Read the model definition and answer for the solid it produces. Units are mm, in the model's axes. Face numbers are marked on the shaded views. A direction names the side the tool comes from. Round coordinates to 2 decimals unless told otherwise and drop trailing zeros. Loops run counter-clockwise (first coordinate to the right, second up) from the corner with the lowest first, then second, coordinate; pieces in that order, holes last. Notation, with made-up numbers: M -5.5,47 L 23.5,47 A23 cw 23.5,78 Z; hole C 44.25,52.25 d5. An arc over 180 degrees is marked long. Write each question's results on one line, items separated by ' | '.
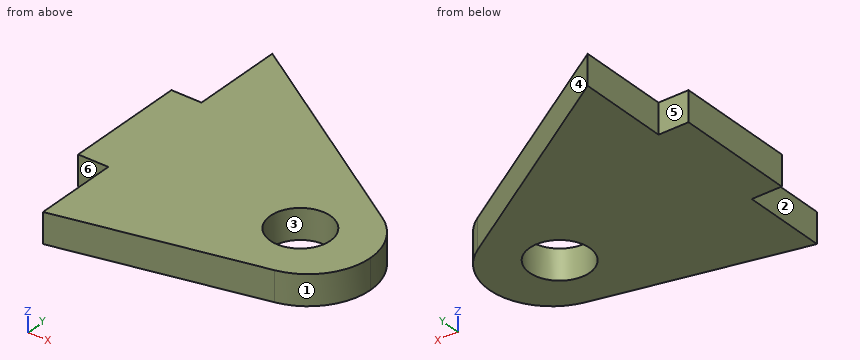
from build123d import *

# Parameters (mm, degrees)
SKETCH1_W                   = 68.548183611
SKETCH1_H                   = 64.912098736
BOSS_EXTRUDE1_DEPTH         = 3.175
F_1_4_0_25_DIAMETER_HOLE1_D = 6.35
CUT_EXTRUDE1_DEPTH          = 95.459063428
FILLET1_R                   = 6.604
SKETCH5_W                   = 3.175
SKETCH5_H                   = 12.7
BOSS_EXTRUDE2_DEPTH         = 3.175


with BuildPart() as part:
    # Sketch1 → Boss-Extrude1 (new body)
    with BuildSketch(Plane.XY):
        with Locations((34.274091805, 32.456049368)):
            Rectangle(SKETCH1_W, SKETCH1_H)
    extrude(amount=BOSS_EXTRUDE1_DEPTH)

    # 1/4 (0.25) Diameter Hole1 (through all)
    with Locations(Plane(origin=(0, 0, 0), x_dir=(-1, 0, 0), z_dir=(0, 0, -1))):
        with Locations((-18.542, 44.846098736)):
            Hole(F_1_4_0_25_DIAMETER_HOLE1_D / 2)

    # Sketch4 → Cut-Extrude1 (cut, through all)
    with BuildSketch(Plane(origin=(0, 0, 0), x_dir=(-1, 0, 0), z_dir=(0, 0, -1))):
        Polygon((-26.0096, 48.402098736), (0, 64.912098736), (-68.548183611, 64.912098736), (-68.548183611, 0), (0, 0), (0, 33.670098736), (-26.0096, 39.512098736), align=None)
    extrude(amount=-CUT_EXTRUDE1_DEPTH, mode=Mode.SUBTRACT)

    # Fillet1
    # the kernel refuses this fillet: 6.604 mm, written as the material it takes off along each edge
    with BuildSketch(Plane(origin=(26.0096, 48.402098736, -9.075328034), x_dir=(-0.84427202966114, 0.5359148625778718, 0), z_dir=(0, 0, 1))) as fillet1_piece_1:
        with BuildLine():
            CenterArc((FILLET1_R * 0.549686737352, FILLET1_R), FILLET1_R, 212.405976432, 57.594023568)
            Line((-FILLET1_R * 0.294585292309, FILLET1_R * 0.464085137422), (0, 0))
            Line((0, 0), (FILLET1_R * 0.549686737352, 0))
        make_face()
    extrude(amount=21.325656067, mode=Mode.SUBTRACT)
    with BuildSketch(Plane(origin=(26.0096, 39.512098736, -13.213034706), x_dir=(-0.9756913106586464, -0.21914941547997013, 0), z_dir=(0, 0, 1))) as fillet1_piece_2:
        with BuildLine():
            CenterArc((FILLET1_R * 0.800304948901, -FILLET1_R), FILLET1_R, 90, 77.340921003)
            Line((-FILLET1_R * 0.175386361757, -FILLET1_R * 0.78085058452), (0, 0))
            Line((0, 0), (FILLET1_R * 0.800304948901, 0))
        make_face()
    extrude(amount=29.601069413, mode=Mode.SUBTRACT)

    # Sketch5 → Boss-Extrude2 (add)
    with BuildSketch(Plane(origin=(0, 0, 0), x_dir=(-1, 0, 0), z_dir=(0, 0, -1))):
        with Locations((1.5875, 48.910098736)):
            Rectangle(SKETCH5_W, SKETCH5_H)
    extrude(amount=-BOSS_EXTRUDE2_DEPTH)


solid = part.part
Item 1: The mould has two halves that part along Y. Classify the marked faces 1, 2 and 3: pulls with the +Y half, pulls with the -Y half, needs draft (parallel to the pull), parting line crosses it, or undercut.
Outcome:
face 1: pulls with the -Y half | face 2: needs draft | face 3: undercut
Item 2: The part is cut by section C-C (y = 47). Determine the outline of the cut face in (x, z) (3 decimals), plus the area to 3 significant figures.
Outcome:
outline: M -3.175,0 L 16.209,0 L 16.209,3.175 L -3.175,3.175 Z; M 20.875,0 L 25.622,0 L 25.622,3.175 L 20.875,3.175 Z | area: 76.6 mm2
Item 3: Flat-ended cylindrical pins translate along their axes: pin 1 (1.5 mm diameter, centred on y = 50, z = 2, fed in from +X); pin 2 (1.6 mm diameter, centred on x = -1.5, z = 1.5, fed in from -Y); pin 3 (1 mm diameter, centred on x = 3, z = 0.5, fed in from +Y). Find the tip coordinate at first contact, or state that the pin passes through.
Outcome:
pin 1: stops at x = 24.26 | pin 2: stops at y = 42.56 | pin 3: stops at y = 63.33
Item 4: The part is cut by section D-D (x = 24.25). Determine the outline of the cut face in (y, z) (3 decimals).
Outcome:
outline: M 40.309,0 L 49.26,0 L 49.26,3.175 L 40.309,3.175 Z
Item 5: The part is cut by section B-B (z = 1.55). Determine the outline of the cut face in (x, y) (3 decimals), plus the area to 3 significant figures.
Outcome:
outline: M -3.175,42.56 L 0,42.56 L 0,33.67 L 20.853,38.354 A6.604 ccw 26.01,44.785 A6.604 ccw 22.945,50.348 L 0,64.912 L 0,55.26 L -3.175,55.26 Z; hole C 18.542,44.846 d6.35 | area: 523 mm2
Item 6: For the marked faces 4, 5 and 6, determine the directions among +Z, -Z, +X, -X, +Y, -Y from which every point of the face is accessible in a straight line to the end or side of a thin tool.
Outcome:
face 4: +Z, -Z, +X, +Y | face 5: +Z, -Z, -X, +Y | face 6: +Z, -Z, -X, -Y
Item 7: Straight lines are drawn through the part: line 1 (X direction, y = 42, z = 1.8); line 2 (Y direction, x = 20, z = 1.5); line 3 (Y direction, x = 21, z = 2.2). For each, find the intervals that lie inside material, in ascending order.
Outcome:
line 1: x = 0 to 17.13, 19.95 to 25.39 | line 2: y = 38.16 to 42.03, 47.67 to 52.22 | line 3: y = 38.39 to 42.84, 46.86 to 51.58
Item 8: The part is cut by section A-A (y = 43.5). Determine the outline of the cut face in (x, z) (3 decimals), plus the area to 3 significant figures.
Outcome:
outline: M -3.175,0 L 15.666,0 L 15.666,3.175 L -3.175,3.175 Z; M 21.418,0 L 25.881,0 L 25.881,3.175 L 21.418,3.175 Z | area: 74.0 mm2
